Autodesk Inventor part; units mm, degrees
ref_plane "YZ Plane" through (0, 0, 0) normal (1, 0, 0) x (0, 1, 0)
ref_plane "XZ Plane" through (0, 0, 0) normal (0, 1, 0) x (-1, 0, 0)
ref_plane "XY Plane" through (0, 0, 0) normal (0, 0, 1) x (1, 0, 0)
sketch "Sketch1" plane through (0, 0, 0) normal (0, 0, 1) x (1, 0, 0)
  circle A0 centre (0, 0) radius 76.2
  circle A1 centre (0, 63.5) radius 3.3734
  circle A2 centre (0, 0) radius 38.1
  circle A3 centre (-31.75, 54.9926) radius 3.3734
  circle A4 centre (-54.9926, 31.75) radius 3.3734
  circle A5 centre (-63.5, 0) radius 3.3734
  circle A6 centre (-54.9926, -31.75) radius 3.3734
  circle A7 centre (-31.75, -54.9926) radius 3.3734
  circle A8 centre (0, -63.5) radius 3.3734
  circle A9 centre (31.75, -54.9926) radius 3.3734
  circle A10 centre (54.9926, -31.75) radius 3.3734
  circle A11 centre (63.5, 0) radius 3.3734
  circle A12 centre (54.9926, 31.75) radius 3.3734
  circle A13 centre (31.75, 54.9926) radius 3.3734
  dimension "d0" = 63.5
  dimension "d1" = 152.4
  dimension "d2" = 6.7469
  dimension "d3" = 76.2
  dimension "d6" = 360
extrude "Extrusion1" add sketch "Sketch1" along normal blind 6.35
sketch "Sketch2" plane through (0, 0, 6.35) normal (0, 0, 1) x (1, 0, 0)
  circle A0 centre (0, 0) radius 46.2375
  circle A1 centre (0, 0) radius 52.5875
  dimension "d10" = 92.475
  dimension "d11" = 6.35
extrude "Extrusion2" add sketch "Sketch2" along normal blind 12.7
sketch "Sketch3" plane through (0, 0, 6.35) normal (0, 0, 1) x (1, 0, 0)
  circle A0 centre (0, 63.5) radius 3.3734
  circle A1 centre (-54.9926, 31.75) radius 3.3734
  circle A2 centre (54.9926, -31.75) radius 3.3734
  circle A3 centre (0, -63.5) radius 3.3734
  circle A4 centre (-63.5, 0) radius 3.3734
  circle A5 centre (31.75, 54.9926) radius 3.3734
  circle A6 centre (-31.75, 54.9926) radius 3.3734
  circle A7 centre (54.9926, 31.75) radius 3.3734
  circle A8 centre (-31.75, -54.9926) radius 3.3734
  circle A9 centre (-54.9926, -31.75) radius 3.3734
  circle A10 centre (31.75, -54.9926) radius 3.3734
  circle A11 centre (63.5, 0) radius 3.3734
  circle A12 centre (0, 0) radius 76.2
  circle A13 centre (0, 0) radius 52.5875
extrude "Extrusion3" add sketch "Sketch3" along normal blind 12.7
sketch "Sketch4" plane through (0, 0, 19.05) normal (0, 0, 1) x (1, 0, 0)
  circle A0 centre (0, 63.5) radius 3.3734 construction
  circle A1 centre (0, 63.5) radius 11.1125
  circle A2 centre (-54.9926, 31.75) radius 11.1125
  circle A3 centre (-54.9926, -31.75) radius 11.1125
  circle A4 centre (0, -63.5) radius 11.1125
  circle A5 centre (54.9926, -31.75) radius 11.1125
  circle A6 centre (54.9926, 31.75) radius 11.1125
  point P0 (0, 0)
  dimension "d16" = 22.225
  dimension "d19" = 360
extrude "Extrusion4" cut sketch "Sketch4" against normal blind 6.35
sketch "Sketch5" plane through (0, 0, 0) normal (0, 0, -1) x (-1, 0, 0)
  circle A0 centre (0, 0) radius 76.2
  line L0 (-76.2, 0) -> (-76.2, 127)
  line L1 (-76.2, 127) -> (76.2, 127)
  line L2 (76.2, 127) -> (76.2, 0)
  circle A1 centre (0, 0) radius 76.2
  dimension "d23" = 127
extrude "Extrusion5" add sketch "Sketch5" against normal blind 12.7 contours A0 L0 L1 L2
sketch "Sketch6" plane through (0, 0, 19.05) normal (0, 0, 1) x (1, 0, 0)
  circle A0 centre (-63.5, 114.3) radius 3.3734
  line L0 (-76.2, 127) -> (-76.2, 0)
  line L1 (76.2, 127) -> (-76.2, 127)
  circle A1 centre (-63.5, 88.9) radius 3.3734
  circle A2 centre (-63.5, 63.5) radius 3.3734
  circle A3 centre (-38.1, 114.3) radius 3.3734
  circle A4 centre (-38.1, 88.9) radius 3.3734
  circle A5 centre (-38.1, 63.5) radius 3.3734
  circle A6 centre (-12.7, 114.3) radius 3.3734
  circle A7 centre (-12.7, 88.9) radius 3.3734
  circle A8 centre (-12.7, 63.5) radius 3.3734
  circle A9 centre (12.7, 114.3) radius 3.3734
  circle A10 centre (12.7, 88.9) radius 3.3734
  circle A11 centre (12.7, 63.5) radius 3.3734
  circle A12 centre (38.1, 114.3) radius 3.3734
  circle A13 centre (38.1, 88.9) radius 3.3734
  circle A14 centre (38.1, 63.5) radius 3.3734
  circle A15 centre (63.5, 114.3) radius 3.3734
  circle A16 centre (63.5, 88.9) radius 3.3734
  circle A17 centre (63.5, 63.5) radius 3.3734
  point P0 (0, 0)
  dimension "d26" = 6.7469
  dimension "d27" = 63.5
  dimension "d28" = 114.3
  dimension "d31" = 25.4
  dimension "d34" = 25.4
extrude "Extrusion6" cut sketch "Sketch6" against normal through all contours A0 | A1 | A2 | A3 | A4 | A6 | A7 | A9 | A10 | A12 | A13 | A15 | A16 | A17
properties part number "28521_Bearing_Holder_Shooter"
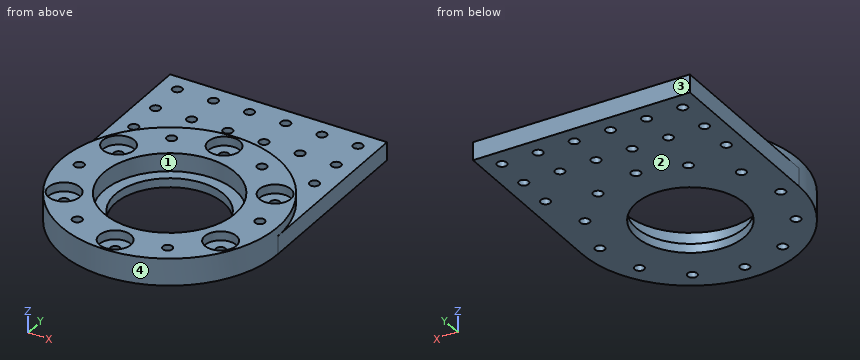
Geometry check sheet. Reference: the model listing, model coordinates, mm. Face numbers are marked on the shaded views. Coordinates: 2 decimals unless noted, no trailing zeros. Write each loop counter-clockwise with the first axis right and the second up, starting at its lowest first coordinate (ties: lowest second). Pieces come first, ordered by that corner, then holes. Notation, with made-up numbers: M 44.5,-22 L 79.5,-22 A22 ccw 79.5,4 Z; hole C -9.75,3.5 d11. An arc over 180 degrees is marked long. One line per item, written item: value. Start each with the question number.
(1) Release check for a two-part mould opening along Y. For the marked faces 1, 2, 3 and 4 record: released by +Y, released by -Y, zero draft, split by the parting line, or undercut.
(2) Sectioned sample at B-B, the plane x = 0. State how many separate pieces and enclosed holes the cut face has, and give its area (3 significant figures).
(3) Depth check by flat-ended pin: pin 1 (13.5 mm diameter, centred on x = -54.99, y = -31.75, fed in from +Z); pin 2 (4 mm diameter, centred on x = 63.5, y = 88.9, fed in from +Z); pin 3 (20 mm diameter, centred on x = 54.99, y = 31.75, fed in from -Z); pin 4 (5 mm diameter, centred on x = -21, z = 7.5, fed in from -Y). Enter the tip coordinate at first touch or a pass-through.
(4) Sectioned sample at A-A, the plane y = 114.3. Enter the section's corners in (x, z).
(5) Sectioned sample at C-C, the plane y = -13. Enter the section's corners in (x, z), and give its area (3 significant figures).
(6) Scan lines: line 1 along Y through (x, z) = (0, 6); line 2 along Y through (x, z) = (0, 15.5); line 3 along Y through (x, z) = (40, 5.75). Record each from-to range of solid material in increasing order. Write a range as [from, to].
Filled sheet:
1. face 1: undercut
1. face 2: zero draft
1. face 3: released by +Y
1. face 4: split by the parting line
2. separate pieces: 4
2. enclosed holes: 0
2. area: 1,440 mm²
3. pin 1: z = 12.7
3. pin 2: through
3. pin 3: z = 0
3. pin 4: y = -73.92
4. outline: M -76.2,0 L -66.87,0 L -66.87,12.7 L -76.2,12.7 Z; M -60.13,0 L -41.47,0 L -41.47,12.7 L -60.13,12.7 Z; M -34.73,0 L -16.07,0 L -16.07,12.7 L -34.73,12.7 Z; M -9.33,0 L 9.33,0 L 9.33,12.7 L -9.33,12.7 Z; M 16.07,0 L 34.73,0 L 34.73,12.7 L 16.07,12.7 Z; M 41.47,0 L 60.13,0 L 60.13,12.7 L 41.47,12.7 Z; M 66.87,0 L 76.2,0 L 76.2,12.7 L 66.87,12.7 Z
5. outline: M -75.08,0 L -35.81,0 L -35.81,6.35 L -44.37,6.35 L -44.37,19.05 L -75.08,19.05 Z; M 35.81,0 L 75.08,0 L 75.08,19.05 L 44.37,19.05 L 44.37,6.35 L 35.81,6.35 Z
5. area: 1,280 mm²
6. line 1: [-76.2, -66.87], [-60.13, -38.1], [38.1, 60.13], [66.87, 127]
6. line 2: [-76.2, -74.61], [-52.39, -46.24], [46.24, 52.39], [74.61, 76.2]
6. line 3: [-64.86, 86.11], [91.69, 111.51], [117.09, 127]
